Source: CAD feature listing. Evaluate the final solid. Frame: model axes, mm. Give positions to 0.01 mm unless a question says otherwise; leave off trailing zeros. Order: outer loops, then holes, each group sorted by start corner. A loop starts at its lowest first (then second) coordinate and runs counter-clockwise, first axis right, second up. Notation, with made-up numbers: M 84,89 L 88,89 A4 cw 88,93 Z; hole C 21.5,83.25 d3. An arc over 180 degrees is marked long. Return JSON: item names as keys, results as strings.
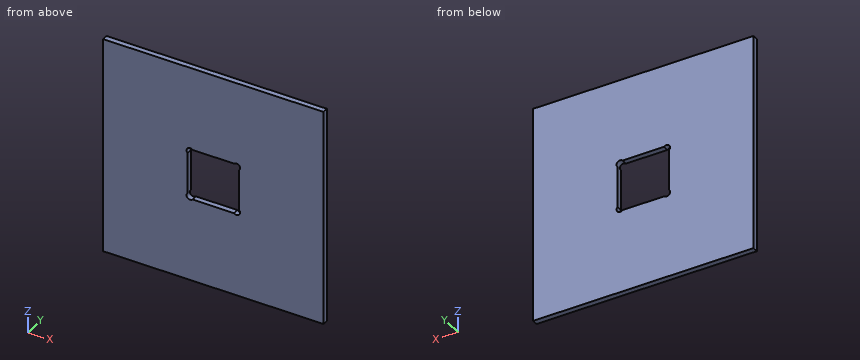
from build123d import *

# Parameters (mm, degrees)
SKETCH_1_W          = 62.64117319
SKETCH_1_H          = 62.64117319
EXTRUDE_1_DEPTH     = 1.6
CUT_EXTRUDE_1_DEPTH = 1.6


with BuildPart() as part:
    # 草图1 → 凸台-拉伸1 (new body)
    with BuildSketch(Plane(origin=(0, 0, 0), x_dir=(1, 0, 0), z_dir=(0, 1, 0))):
        Rectangle(SKETCH_1_W, SKETCH_1_H)
    extrude(amount=EXTRUDE_1_DEPTH)

    # 草图2 → 切除-拉伸1 (cut)
    with BuildSketch(Plane(origin=(0, 1.6, 0), x_dir=(1, 0, 0), z_dir=(0, 1, 0))):
        with BuildLine():
            Line((-5.906373033, 7.320586595), (5.906373033, 7.320586595))
            ThreePointArc((5.906373033, 7.320586595), (7.320586595, 7.320586595), (7.320586595, 5.906373033))
            Line((7.320586595, 5.906373033), (7.320586595, -5.906373033))
            ThreePointArc((7.320586595, -5.906373033), (7.320586595, -7.320586595), (5.906373033, -7.320586595))
            Line((5.906373033, -7.320586595), (-5.906373033, -7.320586595))
            ThreePointArc((-5.906373033, -7.320586595), (-7.320586595, -7.320586595), (-7.320586595, -5.906373033))
            Line((-7.320586595, -5.906373033), (-7.320586595, 5.906373033))
            ThreePointArc((-7.320586595, 5.906373033), (-7.320586595, 7.320586595), (-5.906373033, 7.320586595))
        make_face()
    extrude(amount=-CUT_EXTRUDE_1_DEPTH, mode=Mode.SUBTRACT)


solid = part.part
1. Ray query, probe 1 along Z at (x, y) = (-5.5, 0.15); probe 2 along Z at (x, y) = (-7.5, 0.55). Return the intervals inside material, ascending.
Evaluation:
{"probe 1": "z = -31.32 to -7.32, 7.32 to 31.32", "probe 2": "z = -31.32 to -7.08, -6.15 to 6.15, 7.08 to 31.32"}
2. First-contact query: pin 1 (5 mm diameter, centred on x = -9, z = -8.5, fed in from -Y). Flat tip, straight axial feed; report the tip coordinate or a pass-through.
Evaluation:
{"pin 1": "stops at y = 0"}
3. Section query B-B (y = 0.75). Return loops of the section in (x, z), then the cut area to 3 significant figures.
Evaluation:
{"outline": "M -31.32,-31.32 L 31.32,-31.32 L 31.32,31.32 L -31.32,31.32 Z; hole M -7.32,-5.91 A1 ccw -5.91,-7.32 L 5.91,-7.32 A1 ccw 7.32,-5.91 L 7.32,5.91 A1 ccw 5.91,7.32 L -5.91,7.32 A1 ccw -7.32,5.91 Z", "area": "3,710 mm^2"}
4. Section query A-A (x = 2.5). Return loops of the section in (y, z), then the cut area to 3 significant figures.
Evaluation:
{"outline": "M 0,-31.32 L 1.6,-31.32 L 1.6,-7.32 L 0,-7.32 Z; M 0,7.32 L 1.6,7.32 L 1.6,31.32 L 0,31.32 Z", "area": "76.8 mm^2"}
5. Section query C-C (z = -1). Return loops of the section in (x, y), then the cut area to 3 significant figures.
Evaluation:
{"outline": "M -31.32,0 L -7.32,0 L -7.32,1.6 L -31.32,1.6 Z; M 7.32,0 L 31.32,0 L 31.32,1.6 L 7.32,1.6 Z", "area": "76.8 mm^2"}
